Geometry check sheet. Reference: the model listing, model coordinates, mm. Round coordinates to 2 decimals unless told otherwise and drop trailing zeros. Use one line per item in the form item = value.
Autodesk Inventor part; units mm, degrees
ref_plane "YZ Plane" through (0, 0, 0) normal (1, 0, 0) x (0, 1, 0)
ref_plane "XZ Plane" through (0, 0, 0) normal (0, 1, 0) x (-1, 0, 0)
ref_plane "XY Plane" through (0, 0, 0) normal (0, 0, 1) x (1, 0, 0)
sketch "Sketch1" plane through (0, 0, 0) normal (0, 1, 0) x (-1, 0, 0)
  line L0 (0, 0) -> (-25.4, 0)
  line L1 (-25.4, 0) -> (-25.4, -304.8)
  line L2 (-25.4, -304.8) -> (0, -304.8)
  line L3 (0, -304.8) -> (0, 0)
  line L4 (-12.7, 0) -> (-12.7, -304.8) construction
  line L5 (-12.7, 0) -> (-12.7, -25.4)
  line L6 (-12.7, 0) -> (12.7, 0) construction
  circle A0 centre (-12.7, -25.4) radius 2.3813
  circle A1 centre (-12.7, -38.1) radius 2.3813
  circle A2 centre (-12.7, -50.8) radius 2.3813
  circle A3 centre (-12.7, -63.5) radius 2.3813
  circle A4 centre (-12.7, -76.2) radius 2.3813
  circle A5 centre (-12.7, -88.9) radius 2.3813
  circle A6 centre (-12.7, -101.6) radius 2.3813
  circle A7 centre (-12.7, -114.3) radius 2.3813
  circle A8 centre (-12.7, -127) radius 2.3813
  circle A9 centre (-12.7, -139.7) radius 2.3813
  circle A10 centre (-12.7, -152.4) radius 2.3813
  circle A11 centre (-12.7, -165.1) radius 2.3813
  circle A12 centre (-12.7, -177.8) radius 2.3813
  circle A13 centre (-12.7, -190.5) radius 2.3813
  circle A14 centre (-12.7, -203.2) radius 2.3813
  circle A15 centre (-12.7, -215.9) radius 2.3813
  circle A16 centre (-12.7, -228.6) radius 2.3813
  circle A17 centre (-12.7, -241.3) radius 2.3813
  circle A18 centre (-12.7, -254) radius 2.3813
  circle A19 centre (-12.7, -266.7) radius 2.3813
  circle A20 centre (-12.7, -279.4) radius 2.3813
  circle A21 centre (-12.7, -292.1) radius 2.3813
  dimension "d0" = 25.4
  dimension "d1" = 304.8
  dimension "d2" = 25.4
  dimension "d3" = 90
  dimension "d4" = 4.7625
  dimension "d16" = 12.7
extrude "Extrusion2" add sketch "Sketch1" along normal blind 11.938
properties part number "pincer2.0"
1. Mould release check, pull along Z, two halves, no side actions. Record for faces 1 (the flat face through (13, 6, -304.8)), 2 (the flat face through (25.4, 6, -150)), 3 (the cylindrical face through (13.216, 5.885, -111.975)): released by +Z, released by -Z, zero draft, split by the parting line, or undercut.
Return value:
face_1 = released by -Z
face_2 = zero draft
face_3 = undercut
2. Section check A-A (y = 2.5). Count the separate pieces of the cut face and the enclosed holes in it, then the cut area to 3 significant figures.
Return value:
separate_pieces = 1
enclosed_holes = 22
area = 7,350 mm2
3. Material ranges on line 1 along X through (y, z) = (3, -266.7); line 2 along X through (y, z) = (5.25, -281), recorded low to high.
Return value:
line_1 = 0 to 10.32, 15.08 to 25.4
line_2 = 0 to 10.94, 14.46 to 25.4
